Check sheet for the modelled part. Datum: model origin and axes. Units: mm. Give positions to 0.01 mm unless a question says otherwise; leave off trailing zeros. Order: outer loops, then holes, each group sorted by start corner. A loop starts at its lowest first (then second) coordinate and runs counter-clockwise, first axis right, second up. Notation, with made-up numbers: (57, -23) -> (110, -23) arc R23 ccw to (110, 6) -> close; hole circle Ø11 at (81.5, 40). An arc over 180 degrees is marked (long way). Answer in a Markdown table with one row per item. Add a question column.
(1) Go/stop test with flat-tipped pins: pin 1 (1.5 mm diameter, centred on y = -2, z = 6, fed in from -X); pin 2 (7.5 mm diameter, centred on x = 5.5, y = 1.5, fed in from +Z); pin 3 (4 mm diameter, centred on x = 4, z = 2.5, fed in from -Y). Record where each tip stops, or that it passes through.
(2) Cross-section at C-C (z = 5.5). Record the cut outline in (x, y).
(3) Thickness scan on L1, parallel to Z at x = 4, y = -2.5; L2, parallel to Y at x = 0.25, z = 3.25; L3, parallel to X at y = 3.75, z = 3. Record the ranges inside material, lowest first. Write a range as [from, to].
Autodesk Inventor part; units mm, degrees
ref_plane "YZ Plane" through (0, 0, 0) normal (1, 0, 0) x (0, 1, 0)
ref_plane "XZ Plane" through (0, 0, 0) normal (0, 1, 0) x (-1, 0, 0)
ref_plane "XY Plane" through (0, 0, 0) normal (0, 0, 1) x (1, 0, 0)
sketch "Sketch1" plane through (0, 0, 0) normal (0, 0, 1) x (1, 0, 0)
  circle A0 centre (0, 0) radius 10
  dimension "d0" = 20
extrude "Extrusion1" add sketch "Sketch1" along normal blind 8
sketch "Sketch2" plane through (0, 0, 8) normal (0, 0, 1) x (1, 0, 0)
  circle A0 centre (-3.9419, 3.6305) radius 4.641
  circle A1 centre (5.115, 1.5985) radius 4.641
  circle A2 centre (-1.1732, -5.229) radius 4.641
  circle A3 centre (0, 0) radius 10
  circle A4 centre (0, 0) radius 10
  point P0 (1.9709, -1.8152)
  point P1 (-2.5575, -0.7993)
  point P2 (0.5866, 2.6145)
extrude "Extrusion2" cut sketch "Sketch2" against normal blind 0.01 contours A0 | A1 | A2
properties part number "LED and carclo"
Answer below:
| question | item | result |
|---|---|---|
| 1 | pin 1 | stops at x = -9.92 |
| 1 | pin 2 | stops at z = 7.99 |
| 1 | pin 3 | stops at y = -9.8 |
| 2 | outline | circle Ø20 at (0, 0) |
| 3 | L1 | z = [0, 7.99] |
| 3 | L2 | y = [-10, 10] |
| 3 | L3 | x = [-9.27, 9.27] |
